For this review, use the dimensioned drawing (mm, ordinates from the lowest corner) and the shaded views. Coordinates: 2 decimals unless noted, no trailing zeros. Loops run counter-clockwise (first coordinate to the right, second up) from the corner with the lowest first, then second, coordinate; pieces in that order, holes last. Notation, with made-up numbers: M 52.5,-39.75 L 73.5,-39.75 A8 cw 73.5,-27.75 Z; hole C 3.5,86.25 d10. An arc over 180 degrees is marked long. Write item = value, one per line. Start each with the question number.
Q1. We need section B-B on x = 14.75. Give the boundary of the cut face in (y, z), and give its area (3 significant figures).
Q2. Mouldability with a two-part tool opening along Y and no side actions: class the marked faces 1, 2 and 3 as released by +Y, released by -Y, zero draft, split by the parting line, or undercut.
Q3. Wall thickness on probe 1 along Y at (x, z) = (11.75, 6.5); probe 2 along X at (y, z) = (9.5, 2) (1 decimal); probe 3 along Y at (x, z) = (14.75, 6.25): over which ranges is each line inside the solid? List them lowest first.
Q4. We need section C-C on x = 24.5. Give the boundary of the cut face in (y, z) (1 decimal).
Q5. Clearance check with flat-ended pins moving along their axes: pin 1 Ø6 at (x, y) = (23, 4) entering from -Z; pin 2 Ø5 at (x, y) = (17.5, 13) entering from +Z; pin 3 Ø1.5 at (y, z) = (16, 4.5) entering from +X. State where each tip first meets the part, or that it passes through.
Q6. We need section A-A on z = 2.25. Give the boundary of the cut face in (x, y) (1 decimal), and give its area (3 significant figures).
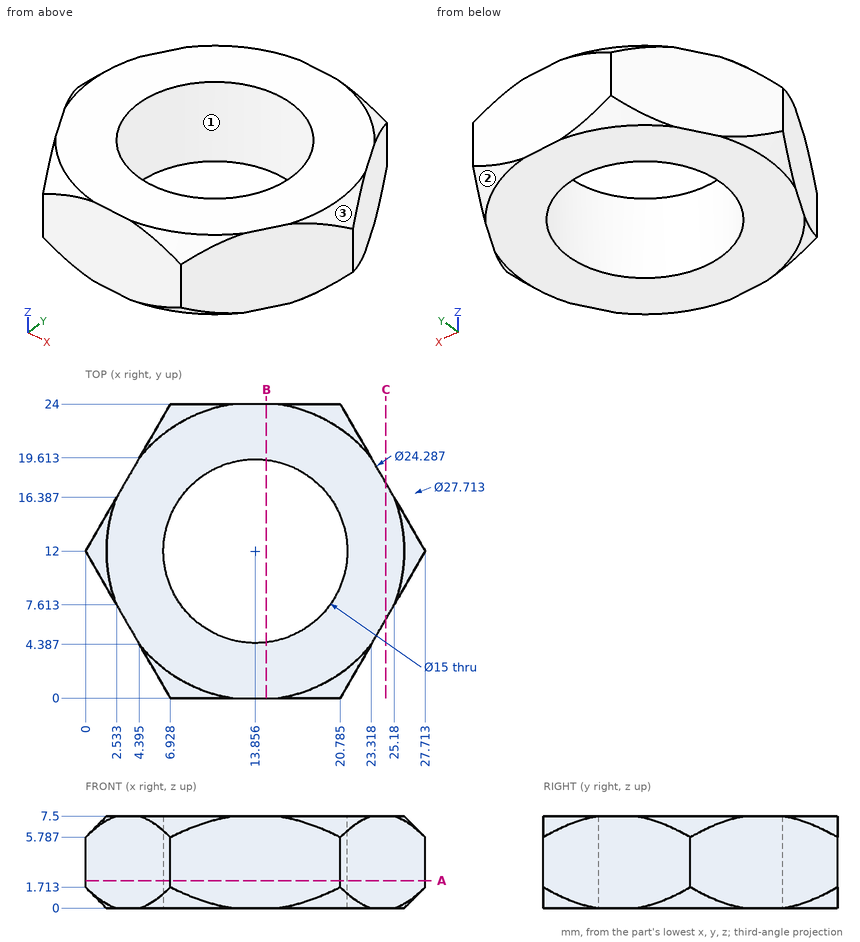
Returned:
q1.outline = M 0,0 L 4.55,0 L 4.55,7.5 L 0,7.5 Z; M 19.45,0 L 24,0 L 24,7.5 L 19.45,7.5 Z
q1.area = 68.3 mm^2
q2.face_1 = undercut
q2.face_2 = released by +Y
q2.face_3 = split by the parting line
q3.probe_1 = 0 to 4.8, 19.2 to 24
q3.probe_2 = 1.4 to 6.8, 20.9 to 26.3
q3.probe_3 = 0 to 4.55, 19.45 to 24
q4.outline = M 6.4,0 L 17.6,0 L 17.6,7.5 L 6.4,7.5 Z
q5.pin_1 = 0
q5.pin_2 = through
q5.pin_3 = 25.84
q6.outline = M 0,12 L 6.9,0 L 20.8,0 L 27.7,12 L 20.8,24 L 6.9,24 Z; hole C 13.9,12 d15
q6.area = 322 mm^2
